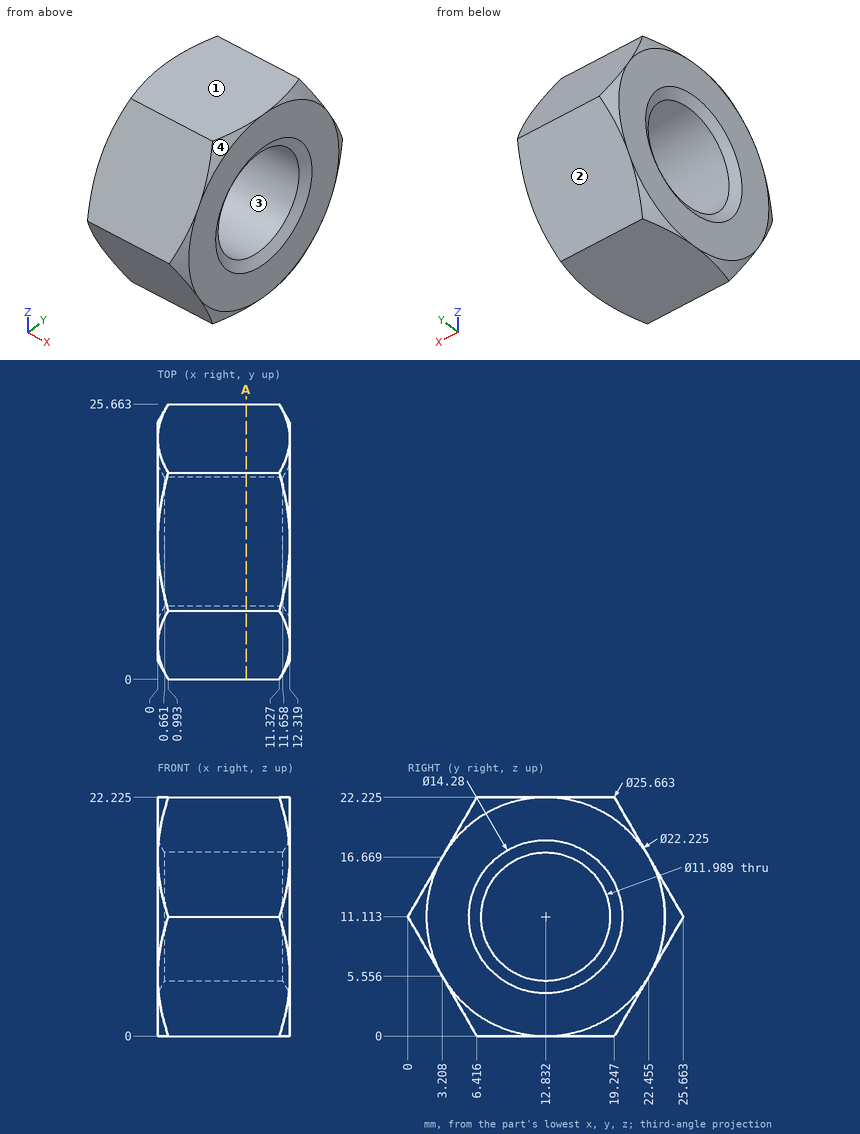
Can you work these out from the drawing? Everything is in mm from the part's minimum corner. Give positions to 0.01 mm unless a question says otherwise; leave off trailing zeros. Order: outer loops, then holes, each group sorted by start corner. A loop starts at its lowest first (then second) coordinate and runs counter-clockwise, first axis right, second up. Notation, with made-up numbers: (68.5, 0.5) -> (89.5, 0.5) arc R23 cw to (89.5, 26.5) -> close; hole circle Ø9 at (-19.75, -14). An arc over 180 degrees is marked (long way). Return JSON: item names as keys, results as strings.
1. Thinking about a two-plate mould opening in Y: for the marked faces 1, 2, 3 and 4, which applies, pulls with the +Y half, pulls with the -Y half, needs draft (parallel to the pull), parting line crosses it, or undercut?
Answer list:
{"face 1": "needs draft", "face 2": "pulls with the +Y half", "face 3": "undercut", "face 4": "pulls with the -Y half"}
2. I need wall thicknesses on line 1 (Z direction, x = 10, y = 11.25) (1 decimal); line 2 (Z direction, x = 11.5, y = 15) (1 decimal); line 3 (Y direction, x = 11, z = 13) (1 decimal). Which ranges of each line are inside material? Lowest first, please. Write a range as from..to.
Answer list:
{"line 1": "z = 0..5.3, 16.9..22.2", "line 2": "z = 0..5.5, 16.7..22.2", "line 3": "y = 1.1..7.1, 18.5..24.6"}
3. Imagine slicing it at A-A on x = 8.25. List the corners of the cut face in (y, z) for me (1 decimal), then the cut area to 3 significant figures.
Answer list:
{"outline": "(0, 11.1) -> (6.4, 0) -> (19.2, 0) -> (25.7, 11.1) -> (19.2, 22.2) -> (6.4, 22.2) -> close; hole circle Ø12 at (12.8, 11.1)", "area": "315 mm2"}
4. For pin 1 Ø1.5 at (x, z) = (1.5, 4) entering from -Y; pin 2 Ø4 at (x, z) = (7, 5.5) entering from -Y (1 decimal); pin 3 Ø1.5 at (x, z) = (3, 2) entering from -Y, each with a flat end and sliding along its axis, tell me the tip position at first contact or that it passes through.
Answer list:
{"pin 1": "stops at y = 3.67", "pin 2": "stops at y = 2.1", "pin 3": "stops at y = 4.83"}
